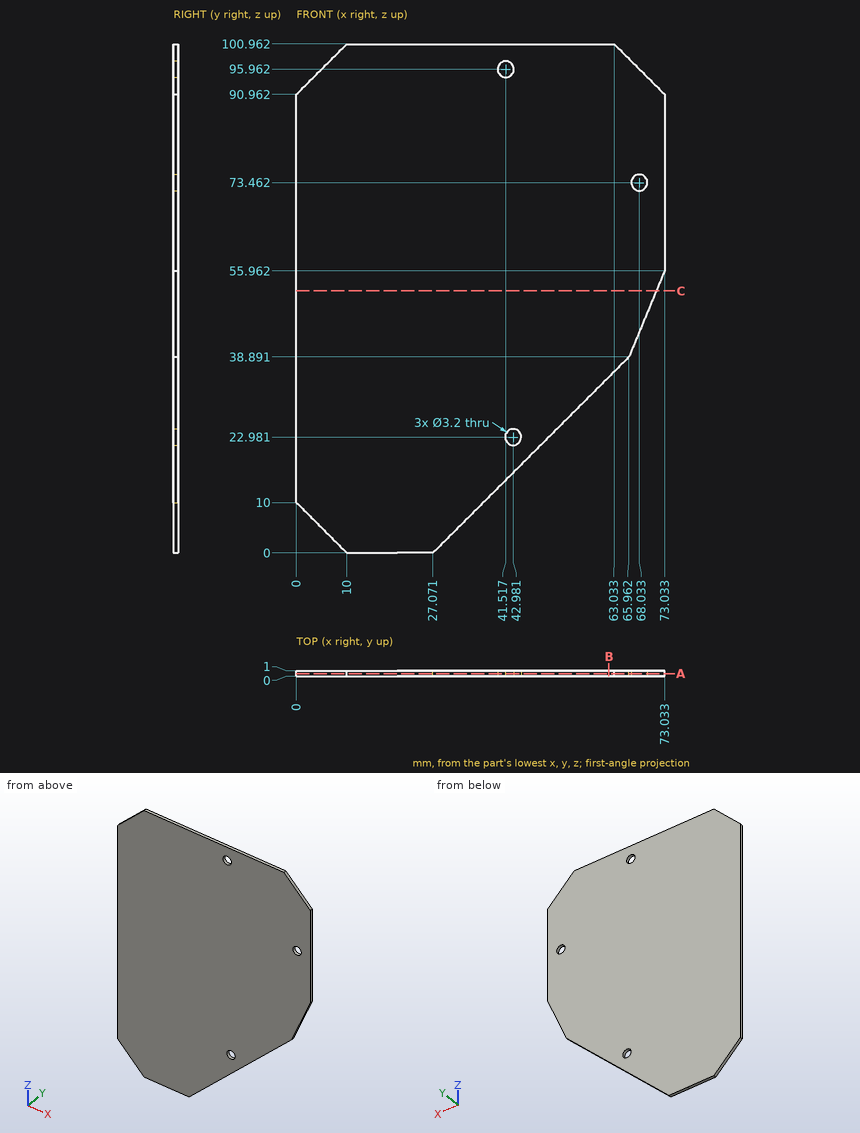
The figure shows three views and two pictorial views of one solid part (mm, origin at its lowest corner). Answer the questions. Round coordinates to 2 decimals unless told otherwise and drop trailing zeros. Order: outer loops, then holes, each group sorted by start corner. A loop starts at its lowest first (then second) coordinate and runs counter-clockwise, first axis right, second up. Notation, with made-up numbers: (53.25, 32) -> (91.25, 32) arc R7 ccw to (91.25, 41) -> close; hole circle Ø2 at (-9.75, -17.75). An arc over 180 degrees is marked (long way). Put each result on its own line as item: value.
Q1. Section C-C, the plane z = 52 is taken. Write down the section's boundary in (x, y).
Results list:
outline: (0, 0) -> (71.39, 0) -> (71.39, 1) -> (0, 1) -> close
Q2. Section A-A, the plane y = 0.45 is taken. Write down the section's boundary in (x, z), and give its area (3 significant figures).
Results list:
outline: (0, 10) -> (10, 0) -> (27.07, 0) -> (65.96, 38.89) -> (73.03, 55.96) -> (73.03, 90.96) -> (63.03, 100.96) -> (10, 100.96) -> (0, 90.96) -> close; hole circle Ø3.2 at (41.52, 95.96); hole circle Ø3.2 at (42.98, 22.98); hole circle Ø3.2 at (68.03, 73.46)
area: 6,110 mm^2
Q3. Consider line 1 along Z through (x, y) = (43.5, 0.3) (1 decimal); line 2 along X through (y, z) = (0.9, 73) (1 decimal); line 3 along Z through (x, y) = (70, 0.2) (1 decimal). Determine where each line is inside the solid, lowest interval first.
Results list:
line 1: 16.4 to 21.5, 24.5 to 101
line 2: 0 to 66.5, 69.6 to 73
line 3: 48.6 to 94
Q4. Section B-B, the plane x = 62 is taken. Write down the section's boundary in (y, z).
Results list:
outline: (0, 34.93) -> (1, 34.93) -> (1, 100.96) -> (0, 100.96) -> close
